```python
from build123d import *

# Parameters (mm, degrees)
SKETCH1_W           = 200
SKETCH1_H           = 100
BOSS_EXTRUDE1_DEPTH = 20
SKETCH2_R           = 27.5
CUT_EXTRUDE1_DEPTH  = 5
SKETCH3_R           = 4
SKETCH3_R_2         = 5.25
CUT_EXTRUDE2_DEPTH  = 16
SKETCH4_R           = 6.5
CUT_EXTRUDE3_DEPTH  = 8
CHAMFER1_SIZE       = 0.5
SKETCH5_R           = 10
CUT_EXTRUDE4_DEPTH  = 21
CHAMFER2_SIZE       = 1
SKETCH7_R           = 11
CUT_EXTRUDE5_DEPTH  = 10
CHAMFER3_SIZE       = 0.5
SKETCH8_R           = 1.5
CUT_EXTRUDE6_DEPTH  = 16


with BuildPart() as part:
    # Sketch1 → Boss-Extrude1 (new body)
    with BuildSketch(Plane.XY):
        Rectangle(SKETCH1_W, SKETCH1_H)
    extrude(amount=-BOSS_EXTRUDE1_DEPTH)

    # Sketch2 → Cut-Extrude1 (cut)
    with BuildSketch(Plane.XY):
        Circle(SKETCH2_R)
    extrude(amount=-CUT_EXTRUDE1_DEPTH, mode=Mode.SUBTRACT)

    # Sketch3 → Cut-Extrude2 (cut, through all)
    with BuildSketch(Plane.XY.offset(-5)):
        with Locations((-20, 0)):
            Circle(SKETCH3_R)
        with Locations((0, 20)):
            Circle(SKETCH3_R)
        with Locations((20, 0)):
            Circle(SKETCH3_R)
        with Locations((0, -20)):
            Circle(SKETCH3_R)
        Circle(SKETCH3_R_2)
    extrude(amount=-CUT_EXTRUDE2_DEPTH, mode=Mode.SUBTRACT)

    # Sketch4 → Cut-Extrude3 (cut)
    with BuildSketch(Plane(origin=(0, 0, -20), x_dir=(-1, 0, 0), z_dir=(0, 0, -1))):
        with Locations((0, 20)):
            Circle(SKETCH4_R)
        with Locations((20, 0)):
            Circle(SKETCH4_R)
        with Locations((0, -20)):
            Circle(SKETCH4_R)
        with Locations((-20, 0)):
            Circle(SKETCH4_R)
    extrude(amount=-CUT_EXTRUDE3_DEPTH, mode=Mode.SUBTRACT)

    # Chamfer1
    chamfer1_edges = [part.edges().sort_by_distance(p)[0] for p in [
        (-27.5, 0, 0),
        (-24, 0, -5),
        (-4, -20, -5),
        (16, 0, -5),
        (-4, 20, -5),
        (6.5, 20, -20),
        (-4, 20, -12),
        (-13.5, 0, -20),
        (-24, 0, -12),
        (6.5, -20, -20),
        (-4, -20, -12),
        (26.5, 0, -20),
        (16, 0, -12),
    ]]
    chamfer(chamfer1_edges, length=CHAMFER1_SIZE)

    # Sketch5 → Cut-Extrude4 (cut, through all)
    with BuildSketch(Plane.XY):
        with Locations((75, 0)):
            Circle(SKETCH5_R)
        with Locations((-75, 0)):
            Circle(SKETCH5_R)
    extrude(amount=-CUT_EXTRUDE4_DEPTH, mode=Mode.SUBTRACT)

    # Chamfer2
    chamfer2_edges = [part.edges().sort_by_distance(p)[0] for p in [
        (65, 0, -20),
        (65, 0, 0),
        (-85, 0, -20),
        (-85, 0, 0),
    ]]
    chamfer(chamfer2_edges, length=CHAMFER2_SIZE)

    # Sketch7 → Cut-Extrude5 (cut)
    with BuildSketch(Plane(origin=(0, 0, -20), x_dir=(-1, 0, 0), z_dir=(0, 0, -1))):
        Circle(SKETCH7_R)
    extrude(amount=-CUT_EXTRUDE5_DEPTH, mode=Mode.SUBTRACT)

    # Chamfer3
    chamfer3_edges = [part.edges().sort_by_distance(p)[0] for p in [
        (11, 0, -10),
    ]]
    chamfer(chamfer3_edges, length=CHAMFER3_SIZE)

    # Sketch8 → Cut-Extrude6 (cut, through all)
    with BuildSketch(Plane.XY.offset(-5)):
        with Locations((0, 7)):
            Circle(SKETCH8_R)
        with Locations((4.949747468, 4.949747468)):
            Circle(SKETCH8_R)
        with Locations((7, 0)):
            Circle(SKETCH8_R)
        with Locations((4.949747468, -4.949747468)):
            Circle(SKETCH8_R)
        with Locations((0, -7)):
            Circle(SKETCH8_R)
        with Locations((-4.949747468, -4.949747468)):
            Circle(SKETCH8_R)
        with Locations((-7, 0)):
            Circle(SKETCH8_R)
        with Locations((-4.949747468, 4.949747468)):
            Circle(SKETCH8_R)
    extrude(amount=-CUT_EXTRUDE6_DEPTH, mode=Mode.SUBTRACT)


solid = part.part
```
The model under review builds one solid part; all positions refer to its coordinate system, in mm. A direction names the side the tool comes from. Coordinates: 2 decimals unless noted, no trailing zeros. Write each loop counter-clockwise with the first axis right and the second up, starting at its lowest first coordinate (ties: lowest second). Pieces come first, ordered by that corner, then holes. Notation, with made-up numbers: (8, 81) - (30, 81) arc R16 cw to (30, 88) - close; hole circle Ø7 at (57, -12). An arc over 180 degrees is marked (long way). Write item = value, one per line.
(1) For P1, Ø3.5, axis at x = 4.95, y = 4.95, coming from the +Z side; P2, Ø4, axis at x = -22, y = 2.5, coming from the -Z side; P3, Ø2.5, axis at x = -4.95, y = 4.95, coming from the +Z side; P4, Ø5, axis at x = 7, y = 0, coming from the -Z side, all flat-tipped, find the tip position at first contact; note any pin that passes through.
Result sheet:
P1 = -5
P2 = -12
P3 = through
P4 = -10
(2) Machinability: for faces 3 (the face through (-1, -50, -10)), 4 (the face through (-13.506, 0.286, -15.802)), which of the approach directions +Z, -Z, +X, -X, +Y, -Y give a long, thin tool a straight path to every point of the face, cutting with its end or side? Answer none if there is none.
Result sheet:
face_3 = +Z, -Z, +X, -X, -Y
face_4 = -Z
(3) For line 1 (Y direction, x = 0, z = -7.3); line 2 (Y direction, x = 0, z = -14.5); line 3 (X direction, y = 2.5, z = -9), list the stretches that pass through material, from the lowest coordinate up. Write a range as [from, to].
Result sheet:
line_1 = [-50, -24], [-16, -8.5], [-5.5, -5.25], [5.25, 5.5], [8.5, 16], [24, 50]
line_2 = [-50, -26.5], [-13.5, -11], [11, 13.5], [26.5, 50]
line_3 = [-100, -84.68], [-65.32, -23.12], [-16.88, -4.62], [4.62, 16.88], [23.12, 65.32], [84.68, 100]
(4) Mouldability with a two-part tool opening along X and no side actions: class faces 1 (the face through (26.494, 0.286, -15.802)), 2 (the face through (-24, 23, 0)) as pulls with the +X half, pulls with the -X half, needs draft (parallel to the pull), parting line crosses it, or undercut.
Result sheet:
face_1 = undercut
face_2 = needs draft
(5) Consider section B-B, the plane z = -15.5. Give the boundary of the cut face in (x, y), then the cut area to 3 significant figures.
Result sheet:
outline = (-100, -50) - (100, -50) - (100, 50) - (-100, 50) - close; hole circle Ø20 at (-75, 0); hole circle Ø13 at (-20, 0); hole circle Ø22 at (0, 0); hole circle Ø13 at (0, -20); hole circle Ø13 at (0, 20); hole circle Ø13 at (20, 0); hole circle Ø20 at (75, 0)
area = 18,500 mm^2
(6) Consider section A-A, the plane x = 75. Give the boundary of the cut face in (y, z), then the cut area to 3 significant figures.
Result sheet:
outline = (-50, -20) - (-11, -20) - (-10, -19) - (-10, -1) - (-11, 0) - (-50, 0) - close; (10, -19) - (11, -20) - (50, -20) - (50, 0) - (11, 0) - (10, -1) - close
area = 1,600 mm^2
